```python
from build123d import *

# Parameters (mm, degrees)
BOSS_EXTRUDE1_DEPTH = 15
REVOLVE1_ANGLE      = 180
SKETCH3_R           = 2.5
CUT_EXTRUDE1_DEPTH  = 37.462309307
CUT_EXTRUDE2_START  = -10
SKETCH4_R           = 4.25
CUT_EXTRUDE2_DEPTH  = 27.462309413
FILLET1_R           = 1
CHAMFER1_SIZE       = 1.529194148
CHAMFER1_SIZE_2     = 1


with BuildPart() as part:
    # Sketch1 → Boss-Extrude1 (new body)
    with BuildSketch(Plane.XY):
        with BuildLine():
            Line((-13.5, 0), (-23.5, 0))
            Line((-23.5, 0), (-23.5, 9.734018716))
            Line((-23.5, 9.734018716), (-16.617009358, 16.617009358))
            ThreePointArc((-16.617009358, 16.617009358), (0, 23.5), (16.617009358, 16.617009358))
            Line((16.617009358, 16.617009358), (23.5, 9.734018716))
            Line((23.5, 9.734018716), (23.5, 0))
            Line((23.5, 0), (13.5, 0))
            ThreePointArc((13.5, 0), (0, 13.5), (-13.5, 0))
        make_face()
    extrude(amount=BOSS_EXTRUDE1_DEPTH)

    # Sketch2 → Revolve1 (revolve)
    with BuildSketch(Plane.XZ):
        with BuildLine():
            Line((-13.5, 15), (-13.5, 0))
            ThreePointArc((-13.5, 0), (-12.348480035, 7.5), (-13.5, 15))
        make_face()
    revolve(axis=Axis((0, 0, 7.5), (0, 0, -1)), revolution_arc=REVOLVE1_ANGLE)

    # Sketch3 → Cut-Extrude1 (cut, through all)
    with BuildSketch(Plane.XZ):
        with Locations((-17.924240018, 7.5)):
            Circle(SKETCH3_R)
        with Locations(Location((17.924240018, 7.5, 0), (0, 0, 121.526459575))):
            Circle(SKETCH3_R)
    extrude(amount=-CUT_EXTRUDE1_DEPTH, mode=Mode.SUBTRACT)

    # Sketch4 → Cut-Extrude2 (cut, through all)
    with BuildSketch(Plane.XZ.offset(CUT_EXTRUDE2_START)):
        with Locations((-17.924240018, 7.5)):
            Circle(SKETCH4_R)
        with Locations(Location((17.924240018, 7.5, 0), (0, 0, 252.086328454))):
            Circle(SKETCH4_R)
    extrude(amount=-CUT_EXTRUDE2_DEPTH, mode=Mode.SUBTRACT)

    # Fillet1
    fillet1_edges = [part.edges().sort_by_distance(p)[0] for p in [
        (23.5, 9.734018716, 7.5),
        (23.5, 0, 7.5),
        (-23.5, 0, 7.5),
        (-23.5, 9.734018716, 7.5),
    ]]
    fillet(fillet1_edges, radius=FILLET1_R)

    # Chamfer1
    # the kernel refuses this chamfer: 1.529194148, 1 mm, written as the material it takes off along each edge
    with BuildSketch(Plane(origin=(0, 0, 15), x_dir=(0.9571659368895994, -0.2895399268810014, 0), z_dir=(-0.2895399268810014, -0.9571659368895994, 0))) as chamfer1_piece_1:
        with BuildLine():
            Line((13.224132078, -0.941354132), (13.5 + CHAMFER1_SIZE, 0))
            Line((13.5 + CHAMFER1_SIZE, 0), (13.5, 0))
            ThreePointArc((13.5, 0), (13.351499892, -0.489654504), (13.224132078, -0.941354132))
        make_face()
    revolve(axis=Axis((0, 0, 15), (0, 0, 1)), revolution_arc=213.660828251, mode=Mode.SUBTRACT)
    with BuildSketch(Plane(origin=(0, 0, 0), x_dir=(0.9613944909393555, -0.27517382286739694, 0), z_dir=(-0.27517382286739694, -0.9613944909393555, 0))) as chamfer1_piece_2:
        with BuildLine():
            Line((13.5 + CHAMFER1_SIZE_2, 0), (13.105478256, 1.394521744))
            ThreePointArc((13.105478256, 1.394521744), (13.285379501, 0.720089037), (13.5, 0))
            Line((13.5, 0), (13.5 + CHAMFER1_SIZE_2, 0))
        make_face()
    revolve(axis=Axis((0, 0, 0), (0, 0, 1)), revolution_arc=211.944746271, mode=Mode.SUBTRACT)
    # the kernel refuses this chamfer: 1.529194148, 1 mm, written as the material it takes off along each edge
    with BuildSketch(Plane(origin=(-23.207106781, 10.026911935, 0), x_dir=(0.7071067811865477, -0.7071067811865475, 0), z_dir=(0.7071067811865475, 0.7071067811865477, 0)), Plane(origin=(16.617009358, 16.617009358, 0), x_dir=(-0.7071067811865477, -0.7071067811865475, 0), z_dir=(0.7071067811865475, -0.7071067811865477, 0))) as chamfer1_2_piece_1:
        Polygon((CHAMFER1_SIZE_2, 0), (0, -CHAMFER1_SIZE_2), (0, 0), align=None)
    extrude(amount=9.319805153, mode=Mode.SUBTRACT)
    with BuildSketch(Plane(origin=(0, 0, 0), x_dir=(-0.7071067811865478, 0.7071067811865472, 0), z_dir=(-0.7071067811865472, -0.7071067811865478, 0))) as chamfer1_2_piece_2:
        Polygon((23.5 - CHAMFER1_SIZE_2, 0), (23.5, -CHAMFER1_SIZE_2), (23.5, 0), align=None)
    revolve(axis=Axis((0, 0, 0), (0, 0, -1)), revolution_arc=90, mode=Mode.SUBTRACT)
    with BuildSketch(Plane(origin=(-23.207106781, 10.026911935, 15), x_dir=(0.7071067811865477, -0.7071067811865475, 0), z_dir=(0.7071067811865475, 0.7071067811865477, 0)), Plane(origin=(16.617009358, 16.617009358, 15), x_dir=(-0.7071067811865477, -0.7071067811865475, 0), z_dir=(0.7071067811865475, -0.7071067811865477, 0))) as chamfer1_2_piece_3:
        Polygon((CHAMFER1_SIZE_2, 0), (0, CHAMFER1_SIZE_2), (0, 0), align=None)
    extrude(amount=9.319805153, mode=Mode.SUBTRACT)
    with BuildSketch(Plane(origin=(22.5, 0, 15), x_dir=(0, 1, 0), z_dir=(-1, 0, 0))) as chamfer1_2_piece_4:
        Polygon((CHAMFER1_SIZE_2, 0), (0, CHAMFER1_SIZE_2), (0, 0), align=None)
    extrude(amount=10.04248884, mode=Mode.SUBTRACT)
    with BuildSketch(Plane(origin=(23.5, 9.319805153, 0), x_dir=(-1, 0, 0), z_dir=(0, -1, 0)), Plane(origin=(-23.5, 1, 0), x_dir=(1, 0, 0), z_dir=(0, 1, 0))) as chamfer1_2_piece_5:
        Polygon((CHAMFER1_SIZE_2, 0), (0, -CHAMFER1_SIZE_2), (0, 0), align=None)
    extrude(amount=8.319805153, mode=Mode.SUBTRACT)
    with BuildSketch(Plane(origin=(23.5, 9.319805153, 15), x_dir=(-1, 0, 0), z_dir=(0, -1, 0)), Plane(origin=(-23.5, 1, 15), x_dir=(1, 0, 0), z_dir=(0, 1, 0))) as chamfer1_2_piece_6:
        Polygon((CHAMFER1_SIZE_2, 0), (0, CHAMFER1_SIZE_2), (0, 0), align=None)
    extrude(amount=8.319805153, mode=Mode.SUBTRACT)
    with BuildSketch(Plane(origin=(-11.928317012, 0, 0), x_dir=(0, 0, 1), z_dir=(-1, 0, 0))) as chamfer1_2_piece_7:
        Polygon((CHAMFER1_SIZE_2, 0), (0, CHAMFER1_SIZE_2), (0, 0), align=None)
    extrude(amount=10.571682988, mode=Mode.SUBTRACT)
    with BuildSketch(Plane(origin=(-22.5, 1, 0), x_dir=(0, -1, 0), z_dir=(1, 0, 0))) as chamfer1_2_piece_8:
        Polygon((1 - CHAMFER1_SIZE_2, 0), (1, -CHAMFER1_SIZE_2), (1, 0), align=None)
    revolve(axis=Axis((-22.5, 1, 0), (0, 0, -1)), revolution_arc=90, mode=Mode.SUBTRACT)
    with BuildSketch(Plane(origin=(-22.5, 9.319805153, 0), x_dir=(-1, 0, 0), z_dir=(0, -1, 0))) as chamfer1_2_piece_9:
        Polygon((1 - CHAMFER1_SIZE_2, 0), (1, -CHAMFER1_SIZE_2), (1, 0), align=None)
    revolve(axis=Axis((-22.5, 9.319805153, 0), (0, 0, -1)), revolution_arc=45, mode=Mode.SUBTRACT)
    with BuildSketch(Plane(origin=(22.5, 9.319805153, 0), x_dir=(0.7071067811865458, 0.7071067811865493, 0), z_dir=(-0.7071067811865493, 0.7071067811865458, 0))) as chamfer1_2_piece_10:
        Polygon((1 - CHAMFER1_SIZE_2, 0), (1, -CHAMFER1_SIZE_2), (1, 0), align=None)
    revolve(axis=Axis((22.5, 9.319805153, 0), (0, 0, -1)), revolution_arc=45, mode=Mode.SUBTRACT)
    with BuildSketch(Plane(origin=(22.5, 1, 0), x_dir=(1, 0, 0), z_dir=(0, 1, 0))) as chamfer1_2_piece_11:
        Polygon((1 - CHAMFER1_SIZE_2, 0), (1, -CHAMFER1_SIZE_2), (1, 0), align=None)
    revolve(axis=Axis((22.5, 1, 0), (0, 0, -1)), revolution_arc=90, mode=Mode.SUBTRACT)
    with BuildSketch(Plane(origin=(-12.45751116, 0, 15), x_dir=(0, 0, -1), z_dir=(-1, 0, 0))) as chamfer1_2_piece_12:
        Polygon((CHAMFER1_SIZE_2, 0), (0, -CHAMFER1_SIZE_2), (0, 0), align=None)
    extrude(amount=10.04248884, mode=Mode.SUBTRACT)
    with BuildSketch(Plane(origin=(-22.5, 1, 15), x_dir=(0, -1, 0), z_dir=(1, 0, 0))) as chamfer1_2_piece_13:
        Polygon((1, CHAMFER1_SIZE_2), (1 - CHAMFER1_SIZE_2, 0), (1, 0), align=None)
    revolve(axis=Axis((-22.5, 1, 15), (0, 0, -1)), revolution_arc=90, mode=Mode.SUBTRACT)
    with BuildSketch(Plane(origin=(-22.5, 9.319805153, 15), x_dir=(-1, 0, 0), z_dir=(0, -1, 0))) as chamfer1_2_piece_14:
        Polygon((1 - CHAMFER1_SIZE_2, 0), (1, CHAMFER1_SIZE_2), (1, 0), align=None)
    revolve(axis=Axis((-22.5, 9.319805153, 15), (0, 0, -1)), revolution_arc=45, mode=Mode.SUBTRACT)
    with BuildSketch(Plane(origin=(22.5, 9.319805153, 15), x_dir=(0.7071067811865458, 0.7071067811865493, 0), z_dir=(-0.7071067811865493, 0.7071067811865458, 0))) as chamfer1_2_piece_15:
        Polygon((1 - CHAMFER1_SIZE_2, 0), (1, CHAMFER1_SIZE_2), (1, 0), align=None)
    revolve(axis=Axis((22.5, 9.319805153, 15), (0, 0, -1)), revolution_arc=45, mode=Mode.SUBTRACT)
    with BuildSketch(Plane(origin=(22.5, 1, 15), x_dir=(1, 0, 0), z_dir=(0, 1, 0))) as chamfer1_2_piece_16:
        Polygon((1 - CHAMFER1_SIZE_2, 0), (1, CHAMFER1_SIZE_2), (1, 0), align=None)
    revolve(axis=Axis((22.5, 1, 15), (0, 0, -1)), revolution_arc=90, mode=Mode.SUBTRACT)
    with BuildSketch(Plane(origin=(0, 0, 15), x_dir=(-0.7071067811865478, 0.7071067811865472, 0), z_dir=(-0.7071067811865472, -0.7071067811865478, 0))) as chamfer1_2_piece_17:
        Polygon((23.5 - CHAMFER1_SIZE_2, 0), (23.5, CHAMFER1_SIZE_2), (23.5, 0), align=None)
    revolve(axis=Axis((0, 0, 15), (0, 0, -1)), revolution_arc=90, mode=Mode.SUBTRACT)
    with BuildSketch(Plane(origin=(22.5, 0, 0), x_dir=(0, 1, 0), z_dir=(-1, 0, 0))) as chamfer1_2_piece_18:
        Polygon((CHAMFER1_SIZE_2, 0), (0, -CHAMFER1_SIZE_2), (0, 0), align=None)
    extrude(amount=10.571682988, mode=Mode.SUBTRACT)


solid = part.part
```
Build history of the part. All positions in model axes, mm. A direction names the side the tool comes from. Give positions to 0.01 mm unless a question says otherwise; leave off trailing zeros. Loops run counter-clockwise (first coordinate to the right, second up) from the corner with the lowest first, then second, coordinate; pieces in that order, holes last.
1) Band-saw the part on D-D on x = 0. List the corners of the cut face in (y, z), then the cut area to 3 significant figures.
Values follow:
outline: (13.11, 1.39) - (14.5, 0) - (22.5, 0) - (23.5, 1) - (23.5, 14) - (22.5, 15) - (15.03, 15) - (13.22, 14.06) arc R25 ccw to start
area: 159 mm2
2) Band-saw the part on B-B on y = 7.25. State how many separate pieces and enclosed holes the cut face has, then the cut area to 3 significant figures.
Values follow:
separate pieces: 2
enclosed holes: 2
area: 347 mm2
3) Probe line 1 along Y through (x, z) = (14.5, 7); line 2 along Z through (x, y) = (-17.5, 11); line 3 along X through (y, z) = (3, 2). List the from-to ranges inside material, lowest first.
Values follow:
line 1: y = 0 to 10
line 2: z = 0 to 3.27, 11.73 to 15
line 3: x = -23.5 to -12.61, 12.61 to 23.5
4) Band-saw the part on A-A on z = 6. List the corners of the cut face in (x, y).
Values follow:
outline: (-23.5, 1) arc R1 ccw to (-22.5, 0) - (-19.92, 0) - (-19.92, 10) - (-21.9, 10) - (-21.9, 11.33) - (-23.21, 10.03) arc R1 ccw to (-23.5, 9.32) - close; (-15.92, 0) - (-12.39, 0) arc R12.39 cw to (12.39, 0) - (15.92, 0) - (15.92, 10) - (13.95, 10) - (13.95, 18.91) arc R23.5 ccw to (-13.95, 18.91) - (-13.95, 10) - (-15.92, 10) - close; (19.92, 0) - (22.5, 0) arc R1 ccw to (23.5, 1) - (23.5, 9.32) arc R1 ccw to (23.21, 10.03) - (21.9, 11.33) - (21.9, 10) - (19.92, 10) - close
5) 3-axis set-ups, long thin cutter, end or side, ignore diameter. For faces 1 (the face through (-23.5, 5, 7)), 2 (the face through (13.733, 13.48, 6.794)): which of +Z, -Z, +X, -X, +Y, -Y reach the whole face in a straight line?
Values follow:
face 1: +Z, -Z, -X, +Y, -Y
face 2: +Y
6) Two-plate mould, pull along Z, no slides. Class faces 3 (the face through (15, 10, 8)), 4 (the face through (23, 5.2, 0.5)), 5 (the face through (-22.155, 11.079, 5.965)), 6 (the face through (-22.8, 0.6, 14.5)): released by +Z, released by -Z, zero draft, split by the parting line, or undercut.
Values follow:
face 3: undercut
face 4: released by -Z
face 5: zero draft
face 6: released by +Z
7) Band-saw the part on C-C on z = 2.25. List the corners of the cut face in (x, y), then the cut area to 3 significant figures.
Values follow:
outline: (-23.5, 1) arc R1 ccw to (-22.5, 0) - (-12.91, 0) arc R12.91 cw to (12.91, 0) - (22.5, 0) arc R1 ccw to (23.5, 1) - (23.5, 9.32) arc R1 ccw to (23.21, 10.03) - (16.62, 16.62) arc R23.5 ccw to (-16.62, 16.62) - (-23.21, 10.03) arc R1 ccw to (-23.5, 9.32) - close
area: 629 mm2
8) Drop flat-ended pins along their axis: P1, Ø3, axis at x = -17.92, z = 7.5, coming from the -Y side; P2, Ø2.5, axis at x = 16, z = 7.5, coming from the +Y side; P3, Ø4, axis at x = 3.5, z = 5, coming from the +Y side; P4, Ø7, axis at x = -17, z = 6, coming from the +Y side. Give the stop position or say it passes through.
Values follow:
P1: passes through
P2: stops at y = 10
P3: stops at y = 23.45
P4: stops at y = 19.24
